Can you work these out from the drawing? Everything is in mm from the part's minimum corner. A direction names the side the tool comes from. Give positions to 0.01 mm unless a question says otherwise; leave off trailing zeros. Loops run counter-clockwise (first coordinate to the right, second up) from the corner with the lowest first, then second, coordinate; pieces in that order, holes last.
Q1. Will these pins go through, and if not, where does the flat tip stop? P1, Ø1, axis at y = 12.5, z = 10.5, coming from the +X side; P2, Ø0.7, axis at y = 5.5, z = 10.5, coming from the -X side; P3, Ø8, axis at x = 22.5, y = 4, coming from the -Z side.
Q2. For the marked faces 4, 5 and 6, which set-ups out of +Z, -Z, +X, -X, +Y, -Y let a thin tool reach every point of the face, with its end or its side?
Q3. If we section it at A-A (x = 30): Please give me the cut outline in (y, z), plus the area to 3 significant figures.
Q4. If we section it at C-C (z = 7.5): Please give me the cut outline in (x, y), plus the area to 3 significant figures.
Q5. I need wall thicknesses on line 1 (X direction, y = 7.5, z = 10); line 2 (Z direction, x = 7, y = 18.75); line 3 (X direction, y = 6, z = 12.5) (1 decimal). Which ranges of each line are inside material? Lowest first, please.
Q6. If we section it at D-D (z = 5): Please give me the cut outline in (x, y), plus the area to 3 significant figures.
Q7. We'd pull the mould along Z, two halves only. Please class the marked faces 1, 2 and 3: +Z half, -Z half, draft (parallel to the pull), parting line (faces both ways), or undercut.
Q8. If we section it at B-B (y = 11.75): Please give me the cut outline in (x, z), plus the area to 3 significant figures.
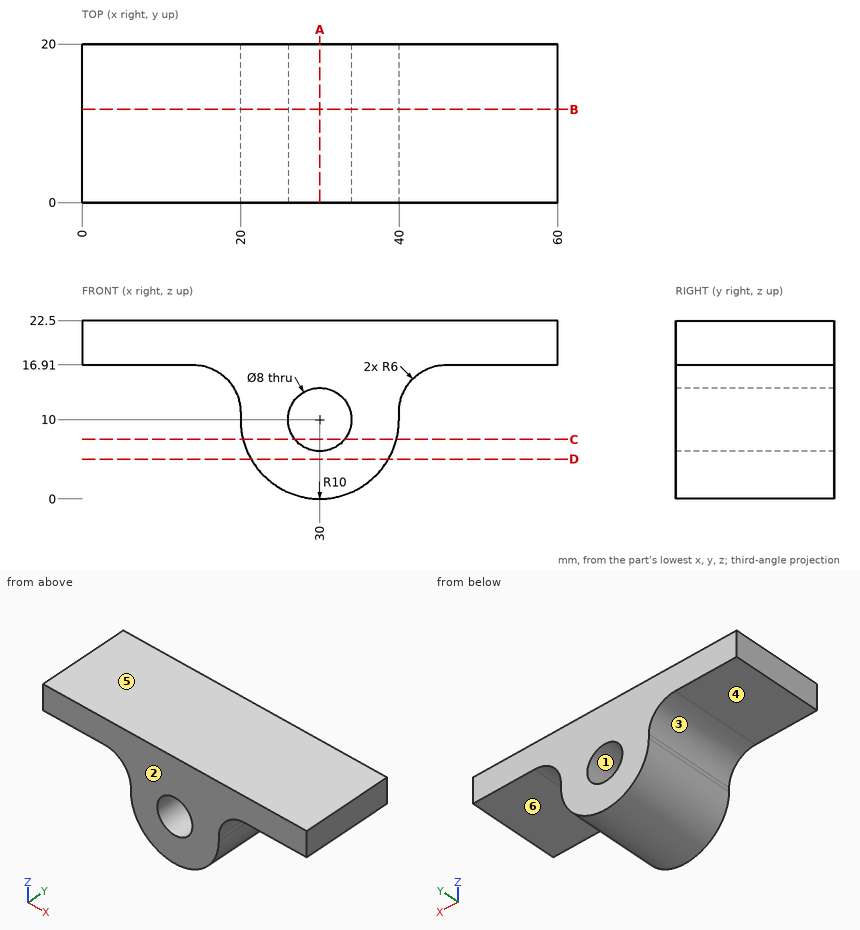
Check sheet entries:
1. P1: stops at x = 40
1. P2: stops at x = 20
1. P3: stops at z = 0.63
2. face 4: -Z, -X, +Y, -Y
2. face 5: +Z, +X, -X, +Y, -Y
2. face 6: -Z, +X, +Y, -Y
3. outline: (0, 0) - (20, 0) - (20, 6) - (0, 6) - close; (0, 14) - (20, 14) - (20, 22.5) - (0, 22.5) - close
3. area: 290 mm2
4. outline: (20.32, 0) - (26.88, 0) - (26.88, 20) - (20.32, 20) - close; (33.12, 0) - (39.68, 0) - (39.68, 20) - (33.12, 20) - close
4. area: 262 mm2
5. line 1: x = 20 to 26, 34 to 40
5. line 2: z = 16.91 to 22.5
5. line 3: x = 19.8 to 26.9, 33.1 to 40.2
6. outline: (21.34, 0) - (38.66, 0) - (38.66, 20) - (21.34, 20) - close
6. area: 346 mm2
7. face 1: undercut
7. face 2: draft
7. face 3: -Z half
8. outline: (0, 16.91) - (14, 16.91) arc R6 cw to (20, 10.91) - (20, 10) arc R10 ccw to (40, 10) - (40, 10.91) arc R6 cw to (46, 16.91) - (60, 16.91) - (60, 22.5) - (0, 22.5) - close; hole circle Ø8 at (30, 10)
8. area: 596 mm2
